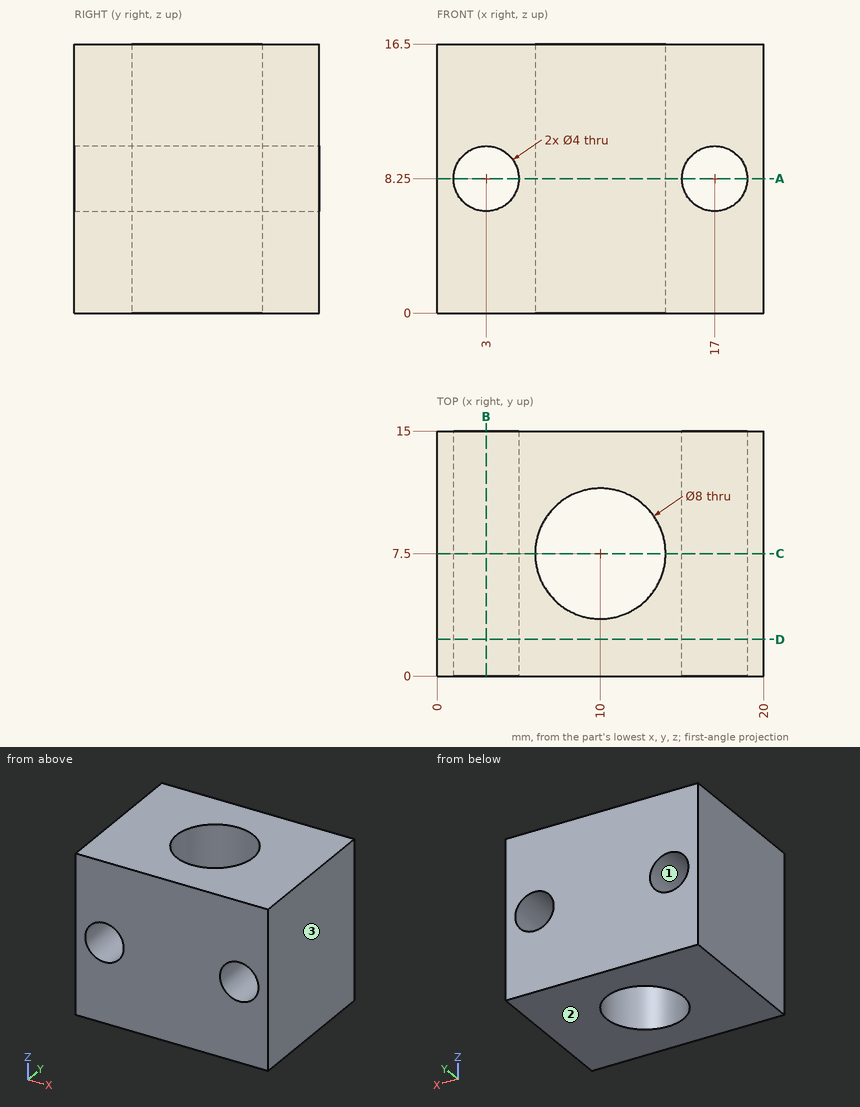
Design review of the part shown in the three views and the two pictorial views. Dimensions are in mm from the part's minimum x, y and z. Round coordinates to 2 decimals unless told otherwise and drop trailing zeros. Write each loop counter-clockwise with the first axis right and the second up, starting at its lowest first coordinate (ties: lowest second). Pieces come first, ordered by that corner, then holes.
Item 1: We need section D-D on y = 2.25. Write out the cut boundary in (x, z).
Item 2: We need section B-B on x = 3. Write out the cut boundary in (y, z).
Item 3: We need section C-C on y = 7.5. Write out the cut boundary in (x, z), and give its area (3 significant figures).
Item 4: For probe 1 along Y at (x, z) = (10, 6.5); probe 2 along X at (y, z) = (7.25, 8.25); probe 3 along X at (y, z) = (4.25, 7), list the stretches that pass through material, from the lowest coordinate up.
Item 5: The part is to be moulded in two halves that separate along Z. For the marked faces 1, 2 and 3, say which applies: +Z half, -Z half, draft (parallel to the pull), parting line (faces both ways), or undercut.
Item 6: We need section A-A on z = 8.25. Write out the cut boundary in (x, y), and give its area (3 significant figures).
Returned:
1. outline: (0, 0) - (20, 0) - (20, 16.5) - (0, 16.5) - close; hole circle Ø4 at (3, 8.25); hole circle Ø4 at (17, 8.25)
2. outline: (0, 0) - (15, 0) - (15, 6.25) - (0, 6.25) - close; (0, 10.25) - (15, 10.25) - (15, 16.5) - (0, 16.5) - close
3. outline: (0, 0) - (6, 0) - (6, 16.5) - (0, 16.5) - close; (14, 0) - (20, 0) - (20, 16.5) - (14, 16.5) - close; hole circle Ø4 at (3, 8.25); hole circle Ø4 at (17, 8.25)
3. area: 173 mm2
4. probe 1: y = 0 to 3.5, 11.5 to 15
4. probe 2: x = 0 to 1, 5 to 6.01, 13.99 to 15, 19 to 20
4. probe 3: x = 0 to 1.44, 4.56 to 7.67, 12.33 to 15.44, 18.56 to 20
5. face 1: undercut
5. face 2: -Z half
5. face 3: draft
6. outline: (0, 0) - (1, 0) - (1, 15) - (0, 15) - close; (5, 0) - (15, 0) - (15, 15) - (5, 15) - close; (19, 0) - (20, 0) - (20, 15) - (19, 15) - close; hole circle Ø8 at (10, 7.5)
6. area: 130 mm2
